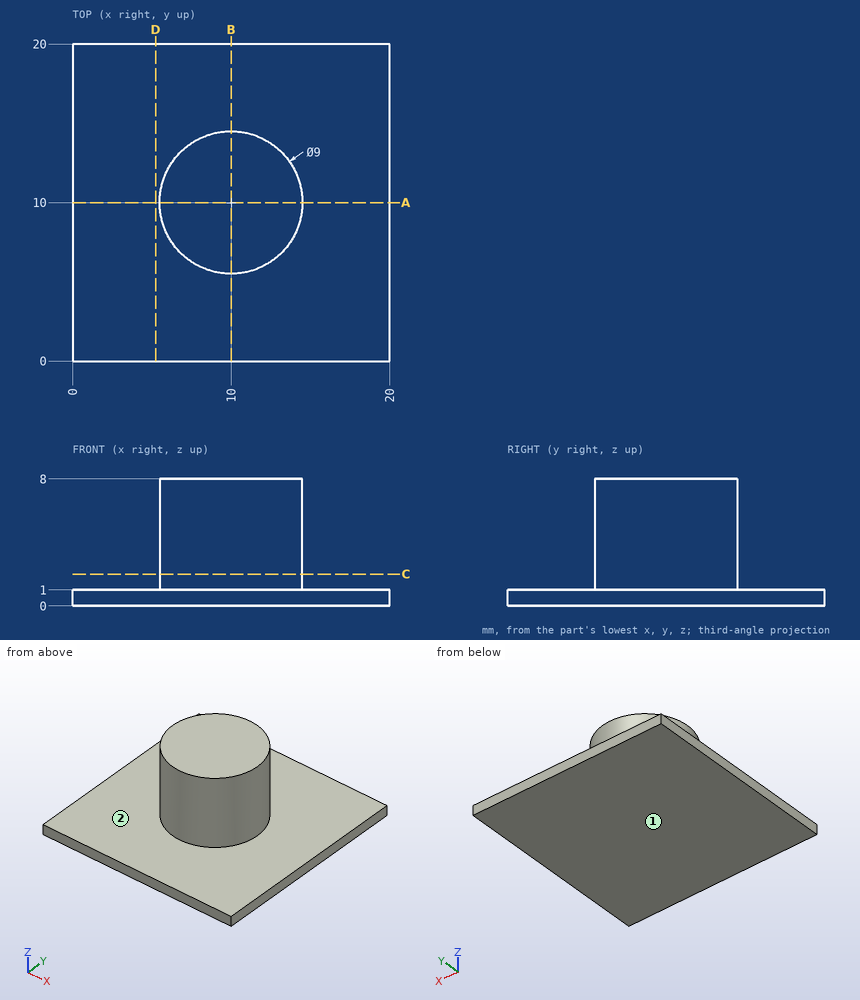
Study the drawing (mm; zero at the part's minimum x, y, z) and answer. A direction names the side the tool comes from. Round coordinates to 2 decimals unless told otherwise and drop trailing zeros. Write each loop counter-clockwise with the first axis right and the second up, starting at its lowest first coordinate (ties: lowest second). Pieces come first, ordered by that corner, then holes. Notation, with made-up numbers: (-15.5, 76) - (10.5, 76) arc R23 cw to (10.5, 101) - close; hole circle Ø5 at (-27, 75). An arc over 180 degrees is marked (long way). Use a Markdown table: item, result. Add a question column.
1. The part is cut by section C-C (z = 2). Write down the section's boundary in (x, y), and give its area (3 significant figures).
2. Consider line 1 (Z direction, x = 17, y = 15.75); line 2 (X direction, y = 14, z = 3.25); line 3 (X direction, y = 6.75, z = 1.25). Determine where each line is inside the solid, lowest interval first.
3. The part is cut by section A-A (y = 10). Write down the section's boundary in (x, z).
4. A tool of negligible diameter and unlimited length cuts with its end or side. For the marked faces 1 and 2, from which of +Z, -Z, +X, -X, +Y, -Y can it reach the whole face along a straight path? Write none if from no direction.
5. Flat-ended cylindrical pins translate along their axes: P1, Ø4, axis at x = 4, z = 4, coming from the -Y side; P2, Ø3, axis at x = 9, z = 6.5, coming from the -Y side; P3, Ø1.5, axis at y = 13.5, z = 5, coming from the +X side. Find the tip coordinate at first contact, or state that the pin passes through.
6. The part is cut by section D-D (x = 5.25). Write down the section's boundary in (y, z).
Reported:
| question | item | result |
|---|---|---|
| 1 | outline | circle Ø9 at (10, 10) |
| 1 | area | 63.6 mm^2 |
| 2 | line 1 | 0 to 1 |
| 2 | line 2 | 7.94 to 12.06 |
| 2 | line 3 | 6.89 to 13.11 |
| 3 | outline | (0, 0) - (20, 0) - (20, 1) - (14.5, 1) - (14.5, 8) - (5.5, 8) - (5.5, 1) - (0, 1) - close |
| 4 | face 1 | -Z, +X, -X, +Y, -Y |
| 4 | face 2 | +Z |
| 5 | P1 | y = 7.94 |
| 5 | P2 | y = 5.5 |
| 5 | P3 | x = 13.56 |
| 6 | outline | (0, 0) - (20, 0) - (20, 1) - (0, 1) - close |
